Read the model definition and answer for the solid it produces. Units are mm, in the model's axes. A direction names the side the tool comes from. Coordinates: 2 decimals unless noted, no trailing zeros. Write each loop counter-clockwise with the first axis right and the second up, starting at its lowest first coordinate (ties: lowest second). Pieces come first, ordered by that corner, then holes. Notation, with made-up numbers: (18.5, 61) -> (32.5, 61) arc R12 cw to (32.5, 81) -> close; hole circle Ø5 at (26, 52). An arc over 180 degrees is marked (long way). One line per item, written item: value. Start each with the question number.
1. Find section B-B, the plane y = 9.25. Write down the section's boundary in (x, z).
2. For a pull along Z with two mould halves and no side action, classify faces 1 (the flat face through (7.94, 4.93, -7.36)), 2 (the flat face through (0, 10, 3)), 3 (the cylindrical face through (-16, 5, 0)) as pulls with the +Z half, pulls with the -Z half, needs draft (parallel to the pull), parting line crosses it, or undercut.
3. Given P1, Ø4, axis at x = -4.5, y = 7, coming from the -Z side; P2, Ø5, axis at y = 8, z = 9, coming from the +X side; P3, Ø3, axis at y = 2.5, z = -5.5, coming from the +X side, each flat-ended and moving along its own axis, determine where each tip first touches the part or whether it passes through.
4. For faces 4 (the flat face through (0, 2, 0)), 5 (the flat face through (-2.474, 4.93, 10.636)), 6 (the flat face through (-10.448, 4.93, 3.176)), determine the directions among +Z, -Z, +X, -X, +Y, -Y from which every point of the face is accessible in a straight line to the end or side of a thin tool.
5. Find section A-A, the plane z = 9.5. Write down the section's boundary in (x, y), and give its area (3 significant figures).
6. Consider line 1 along X through (y, z) = (4.75, 0.75); line 2 along X through (y, z) = (2.75, -9.25); line 3 along X through (y, z) = (7.5, 7.5). Determine where each line is inside the solid, lowest interval first.
7. Find section D-D, the plane x = 13.5. Write down the section's boundary in (y, z).
```python
from build123d import *

# Parameters (mm, degrees)
BOSS_EXTRUDE1_DEPTH = 10
CUT_EXTRUDE1_DEPTH  = 6
SKETCH3_R           = 6
CUT_EXTRUDE2_DEPTH  = 2
CHAMFER1_SIZE       = 2


with BuildPart() as part:
    # Sketch1 → Boss-Extrude1 (new body)
    with BuildSketch(Plane(origin=(0, 0, 0), x_dir=(1, 0, 0), z_dir=(0, 1, 0))):
        with BuildLine():
            ThreePointArc((4.87913418, -13.349613461), (8, -13.856406461), (9.121537298, -10.900260879))
            Line((9.121537298, -10.900260879), (6.793934197, -3.922479738))
            Line((6.793934197, -3.922479738), (14.000671478, -2.449352582))
            ThreePointArc((14.000671478, -2.449352582), (16, 0), (14.000671478, 2.449352582))
            Line((14.000671478, 2.449352582), (6.793934197, 3.922479738))
            Line((6.793934197, 3.922479738), (9.121537298, 10.900260879))
            ThreePointArc((9.121537298, 10.900260879), (8, 13.856406461), (4.87913418, 13.349613461))
            Line((4.87913418, 13.349613461), (0, 7.844959475))
            Line((0, 7.844959475), (-4.87913418, 13.349613461))
            ThreePointArc((-4.87913418, 13.349613461), (-8, 13.856406461), (-9.121537298, 10.900260879))
            Line((-9.121537298, 10.900260879), (-6.793934197, 3.922479738))
            Line((-6.793934197, 3.922479738), (-14.000671478, 2.449352582))
            ThreePointArc((-14.000671478, 2.449352582), (-16, 0), (-14.000671478, -2.449352582))
            Line((-14.000671478, -2.449352582), (-6.793934197, -3.922479738))
            Line((-6.793934197, -3.922479738), (-9.121537298, -10.900260879))
            ThreePointArc((-9.121537298, -10.900260879), (-8, -13.856406461), (-4.87913418, -13.349613461))
            Line((-4.87913418, -13.349613461), (0, -7.844959475))
            Line((0, -7.844959475), (4.87913418, -13.349613461))
        make_face()
    extrude(amount=BOSS_EXTRUDE1_DEPTH)

    # Sketch2 → Cut-Extrude1 (cut)
    # profile 1 of 2: a face of its own
    with BuildSketch(Plane(origin=(0, 10, 0), x_dir=(1, 0, 0), z_dir=(0, 1, 0))):
        with BuildLine():
            Line((-1.878163997, -1.65), (-5.5, -1.65))
            Line((-5.5, -1.65), (-5.5, 1.65))
            Line((-5.5, 1.65), (-1.878163997, 1.65))
            ThreePointArc((-1.878163997, 1.65), (0, 2.5), (1.878163997, 1.65))
            Line((1.878163997, 1.65), (5.5, 1.65))
            Line((5.5, 1.65), (5.5, -1.65))
            Line((5.5, -1.65), (1.878163997, -1.65))
            ThreePointArc((1.878163997, -1.65), (0, -2.5), (-1.878163997, -1.65))
        make_face()
        with BuildLine():
            ThreePointArc((1.809005252, 1.5), (0, 2.35), (-1.809005252, 1.5))
            Line((-1.809005252, 1.5), (-5.35, 1.5))
            Line((-5.35, 1.5), (-5.35, -1.5))
            Line((-5.35, -1.5), (-1.809005252, -1.5))
            ThreePointArc((-1.809005252, -1.5), (0, -2.35), (1.809005252, -1.5))
            Line((1.809005252, -1.5), (5.35, -1.5))
            Line((5.35, -1.5), (5.35, 1.5))
            Line((5.35, 1.5), (1.809005252, 1.5))
        make_face(mode=Mode.SUBTRACT)
    # profile 2 of 2: a face of its own
    with BuildSketch(Plane(origin=(0, 10, 0), x_dir=(1, 0, 0), z_dir=(0, 1, 0))):
        with BuildLine():
            Line((5.35, 1.5), (1.809005252, 1.5))
            ThreePointArc((1.809005252, 1.5), (0, 2.35), (-1.809005252, 1.5))
            Line((-1.809005252, 1.5), (-5.35, 1.5))
            Line((-5.35, 1.5), (-5.35, -1.5))
            Line((-5.35, -1.5), (-1.809005252, -1.5))
            ThreePointArc((-1.809005252, -1.5), (0, -2.35), (1.809005252, -1.5))
            Line((1.809005252, -1.5), (5.35, -1.5))
            Line((5.35, -1.5), (5.35, 1.5))
        make_face()
    extrude(amount=-CUT_EXTRUDE1_DEPTH, mode=Mode.SUBTRACT)

    # Sketch3 → Cut-Extrude2 (cut)
    with BuildSketch(Plane.XZ):
        with Locations(Location((0, 0, 0), (0, 0, 270))):
            Circle(SKETCH3_R)
    extrude(amount=-CUT_EXTRUDE2_DEPTH, mode=Mode.SUBTRACT)

    # Chamfer1
    chamfer1_edges = [part.edges().sort_by_distance(p)[0] for p in [
        (0, 2, 6),
    ]]
    chamfer(chamfer1_edges, length=CHAMFER1_SIZE - 0.0001)  # a hair under: the kernel refuses the full size


solid = part.part
```
Answer block:
1. outline: (-14, -2.45) -> (-6.79, -3.92) -> (-9.12, -10.9) arc R2.5 ccw to (-4.88, -13.35) -> (0, -7.84) -> (4.88, -13.35) arc R2.5 ccw to (9.12, -10.9) -> (6.79, -3.92) -> (14, -2.45) arc R2.5 ccw to (14, 2.45) -> (6.79, 3.92) -> (9.12, 10.9) arc R2.5 ccw to (4.88, 13.35) -> (0, 7.84) -> (-4.88, 13.35) arc R2.5 ccw to (-9.12, 10.9) -> (-6.79, 3.92) -> (-14, 2.45) arc R2.5 ccw to start; hole (-5.5, -1.65) -> (-1.88, -1.65) arc R2.5 ccw to (1.88, -1.65) -> (5.5, -1.65) -> (5.5, 1.65) -> (1.88, 1.65) arc R2.5 ccw to (-1.88, 1.65) -> (-5.5, 1.65) -> close
2. face 1: undercut
2. face 2: needs draft
2. face 3: parting line crosses it
3. P1: stops at z = -14.18
3. P2: stops at x = 9.24
3. P3: stops at x = 7.82
4. face 4: -Y
4. face 5: +Z, +Y, -Y
4. face 6: -X, +Y, -Y
5. outline: (-8.65, 0) -> (-1.47, 0) -> (-1.47, 10) -> (-8.65, 10) -> close; (1.47, 0) -> (8.65, 0) -> (8.65, 10) -> (1.47, 10) -> close
5. area: 144 mm2
6. line 1: x = -15.88 to -5.5, 5.5 to 15.88
6. line 2: x = -8.57 to -1.25, 1.25 to 8.57
6. line 3: x = -7.99 to 7.99
7. outline: (0, -2.55) -> (10, -2.55) -> (10, 2.55) -> (0, 2.55) -> close
